Verification items for this drawing (mm, ordinates from the low corner). A direction names the side the tool comes from. Coordinates: 2 decimals unless noted, no trailing zeros. Order: outer loops, then holes, each group sorted by start corner. A loop starts at its lowest first (then second) coordinate and runs counter-clockwise, first axis right, second up. Notation, with made-up numbers: M 5.5,-27.75 L 9.5,-27.75 A30 ccw 9.5,3.25 Z; hole C -37.75,60.5 d4. An arc over 180 degrees is marked long. Answer as a JSON object with one key per item and string values. Group by question number.
(1) Cross-section at D-D (y = 9.5). Enter the section's corners in (x, z).
(2) Access from +Z, -Z, +X, -X, +Y, -Y to the whole of each face (thin tool, end or side, straight path). Record for the marked faces 1, 2, 3, 4 and 5.
(3) Material ranges on line 1 (X direction, y = 13.5, z = 16); line 2 (Y direction, x = 22, z = 16); line 3 (X direction, y = 20.25, z = 27.5), recorded low to high.
(4) Cross-section at A-A (x = 19.5). Enter the section's corners in (y, z).
(5) Gauge pin test, flat ends, axial feed: pin 1 Ø7 at (x, z) = (19, 14) entering from -Y; pin 2 Ø12 at (y, z) = (21, 7.5) entering from +X; pin 3 Ø1.2 at (x, z) = (3.5, 28) entering from +Y; pin 4 Ø5 at (y, z) = (10, 24) entering from -X. Record the tip position at first contact, or that the pin passes through.
(6) Cross-section at C-C (z = 25). Enter the section's corners in (x, y).
(7) Cross-section at B-B (y = 16). Enter the section's corners in (x, z) (1 decimal).
(8) Mould release check, pull along X, two halves, no side actions. Record for the marked faces 6, 7 and 8: released by +X, released by -X, zero draft, split by the parting line, or undercut.
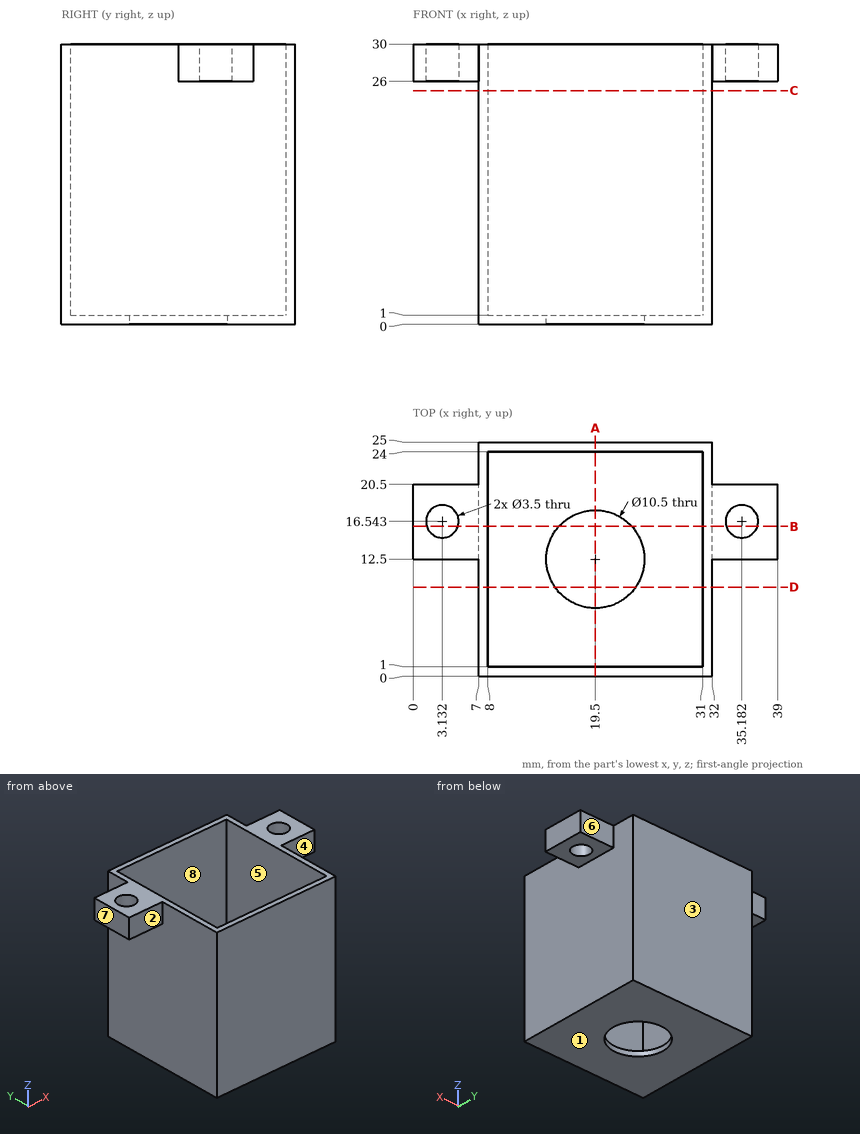
Taken from the geometry:
{
 "1": {"outline": "M 7,0 L 15.19,0 L 15.19,1 L 8,1 L 8,30 L 7,30 Z; M 23.81,0 L 32,0 L 32,30 L 31,30 L 31,1 L 23.81,1 Z"},
 "2": {"face 1": "-Z, +X, -X, +Y, -Y", "face 2": "+Z, -Z, -X, -Y", "face 3": "+Z, -Z, +X, -X, +Y", "face 4": "+Z, -Z, +X, -Y", "face 5": "+Z"},
 "3": {"line 1": "x = 7 to 8, 31 to 32", "line 2": "y = 0 to 1, 24 to 25", "line 3": "x = 0 to 8, 31 to 39"},
 "4": {"outline": "M 0,0 L 7.25,0 L 7.25,1 L 1,1 L 1,30 L 0,30 Z; M 17.75,0 L 25,0 L 25,30 L 24,30 L 24,1 L 17.75,1 Z"},
 "5": {"pin 1": "stops at y = 0", "pin 2": "stops at x = 32", "pin 3": "stops at y = 20.5", "pin 4": "stops at x = 7"},
 "6": {"outline": "M 7,0 L 32,0 L 32,25 L 7,25 Z; hole M 8,1 L 31,1 L 31,24 L 8,24 Z"},
 "7": {"outline": "M 0,26 L 1.5,26 L 1.5,30 L 0,30 Z; M 4.8,26 L 7,26 L 7,0 L 15.6,0 L 15.6,1 L 8,1 L 8,30 L 4.8,30 Z; M 23.4,0 L 32,0 L 32,26 L 33.5,26 L 33.5,30 L 31,30 L 31,1 L 23.4,1 Z; M 36.8,26 L 39,26 L 39,30 L 36.8,30 Z"},
 "8": {"face 6": "zero draft", "face 7": "released by -X", "face 8": "undercut"}
}
